Can you work these out from the drawing? Everything is in mm from the part's minimum corner. A direction names the side the tool comes from. Coordinates: 2 decimals unless noted, no trailing zeros. Order: outer loops, then holes, each group sorted by start corner. A loop starts at its lowest first (then second) coordinate and runs counter-clockwise, first axis right, second up. Notation, with made-up numbers: (-9, -16) -> (2, -16) arc R15 cw to (2, -5) -> close; hole circle Ø10 at (79, 18.5). An arc over 180 degrees is marked (long way). Return JSON: item names as keys, results as strings. Group by question number.
1) If we section it at C-C, the plane x = 46.5: Please give me the cut outline in (y, z) (1 decimal).
2) If I drill on probe 1 along Y at (x, z) = (36, 23); probe 2 along X at (y, z) = (11, 11.5), over which ranges is the centre line in solid material (lowest first)? Write a range as from..to.
3) If we section it at A-A, the plane y = 16.5: Please give me the cut outline in (x, z).
4) If we section it at B-B, the plane z = 27: Please give me the cut outline in (x, y), then the cut area to 3 significant figures.
5) For pin 1 (6 mm diameter, centred on y = 19.5, z = 21.5, fed in from +X); pin 2 (1.5 mm diameter, centred on y = 32, z = 29, fed in from +X); pin 3 (5 mm diameter, centred on x = 44.5, y = 5.5, fed in from +Z), each with a flat end and sliding along its axis, tell me the tip position at first contact or that it passes through.
6) Thinking about a two-plate mould opening in Z: for the marked faces 4, 5, 6 and 7, which applies, +Z half, -Z half, draft (parallel to the pull), parting line (faces both ways), or undercut?
7) If we section it at D-D, the plane x = 27: Please give me the cut outline in (y, z).
8) For the marked faces 1, 2 and 3, which set-ups out of +Z, -Z, +X, -X, +Y, -Y let a thin tool reach every point of the face, with its end or its side?
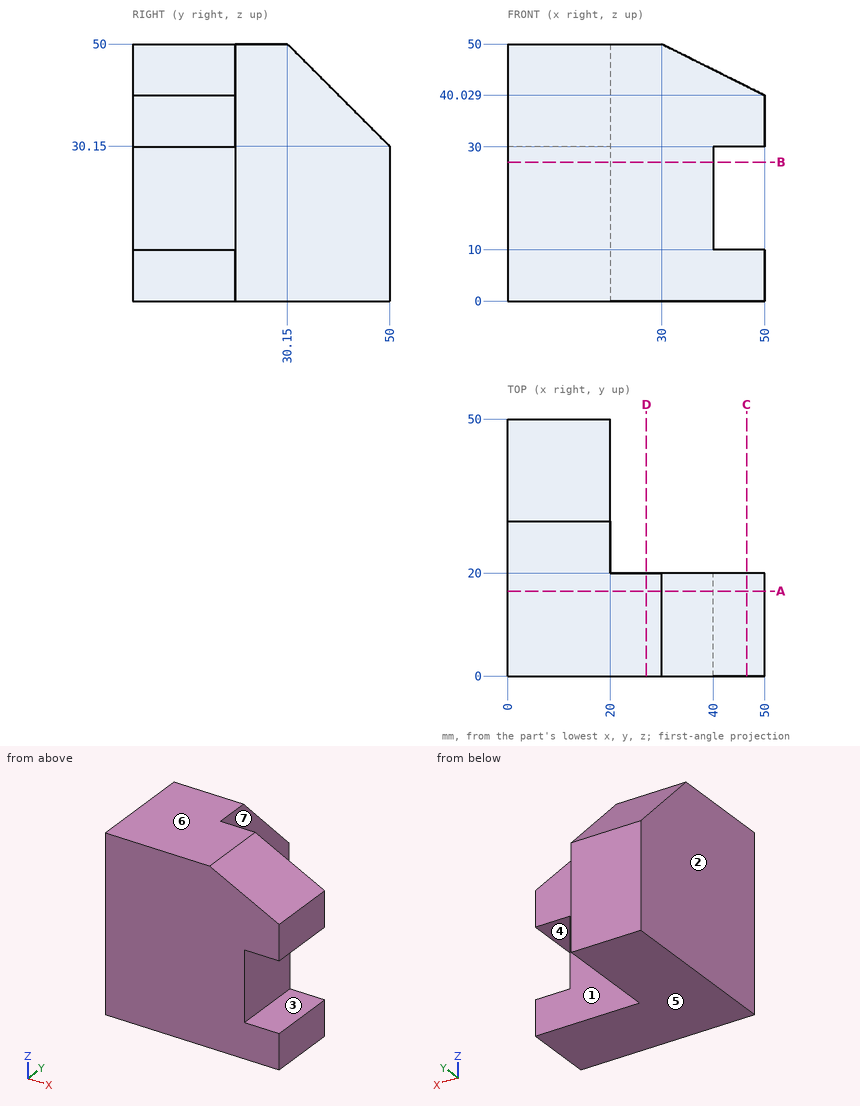
Result sheet:
{
 "1": {"outline": "(0, 0) -> (20, 0) -> (20, 10) -> (0, 10) -> close; (0, 30) -> (20, 30) -> (20, 41.8) -> (0, 41.8) -> close"},
 "2": {"probe 1": "y = 0..20", "probe 2": "x = 0..40"},
 "3": {"outline": "(0, 0) -> (50, 0) -> (50, 10) -> (40, 10) -> (40, 30) -> (50, 30) -> (50, 40.03) -> (30, 50) -> (0, 50) -> close"},
 "4": {"outline": "(0, 0) -> (40, 0) -> (40, 20) -> (20, 20) -> (20, 50) -> (0, 50) -> close", "area": "1,400 mm2"},
 "5": {"pin 1": "stops at x = 40", "pin 2": "stops at x = 20", "pin 3": "stops at z = 44.02"},
 "6": {"face 4": "undercut", "face 5": "-Z half", "face 6": "+Z half", "face 7": "draft"},
 "7": {"outline": "(0, 0) -> (20, 0) -> (20, 50) -> (0, 50) -> close"},
 "8": {"face 1": "+Z, -Z, +X, +Y", "face 2": "+Z, -Z, -X, +Y, -Y", "face 3": "+X, +Y, -Y"}
}
